Here's how the part is built. I have some questions about the finished solid (model axes, mm). Face numbers are marked on the shaded views. A direction names the side the tool comes from. Give positions to 0.01 mm unless a question says otherwise; leave off trailing zeros. Loops run counter-clockwise (first coordinate to the right, second up) from the corner with the lowest first, then second, coordinate; pieces in that order, holes last. Notation, with made-up numbers: (-22.75, -9.75) - (-7.75, -9.75) arc R33 cw to (-7.75, 18.25) - close; hole circle Ø9 at (-25.75, 85.5). An arc over 180 degrees is marked (long way). Use one line per item in the form item = value.
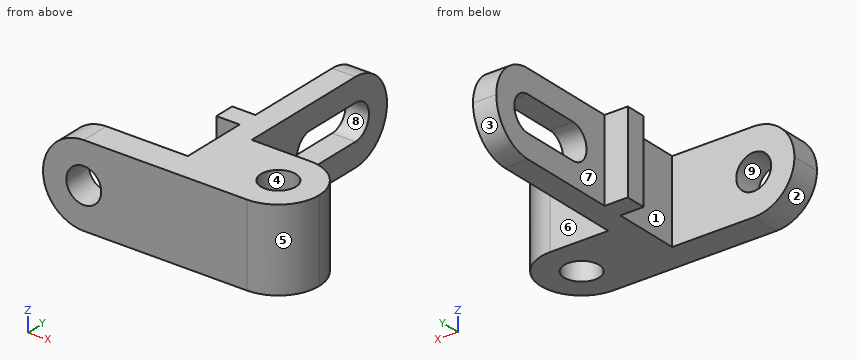
from build123d import *

# Parameters (mm, degrees)
SKETCH2_R           = 6
BOSS_EXTRUDE1_DEPTH = 14
CUT_EXTRUDE1_DEPTH  = 8
SKETCH4_R           = 6
CUT_EXTRUDE2_DEPTH  = 10
FILLET1_R           = 14


with BuildPart() as part:
    # Sketch2 → Boss-Extrude1 (new, symmetric)
    with BuildSketch(Plane.XY):
        Polygon((0, 0), (0, 28), (-34, 28), (-34, 88), (-42, 88), (-42, 40), (-50, 40), (-50, 33), (-42, 33), (-42, 10), (-84, 10), (-84, 0), align=None)
        with Locations((-14, 14)):
            Circle(SKETCH2_R, mode=Mode.SUBTRACT)
    extrude(amount=BOSS_EXTRUDE1_DEPTH, both=True)

    # Sketch3 → Cut-Extrude1 (cut)
    with BuildSketch(Plane(origin=(-34, 0, 0), x_dir=(0, 0, -1), z_dir=(1, 0, 0))):
        with BuildLine():
            Line((-6, 54), (-6, 74))
            ThreePointArc((-6, 74), (0, 80), (6, 74))
            Line((6, 74), (6, 54))
            ThreePointArc((6, 54), (0, 48), (-6, 54))
        make_face()
    extrude(amount=-CUT_EXTRUDE1_DEPTH, mode=Mode.SUBTRACT)

    # Sketch4 → Cut-Extrude2 (cut)
    with BuildSketch(Plane(origin=(0, 10, 0), x_dir=(1, 0, 0), z_dir=(0, 1, 0))):
        with Locations(Location((-70, 0, 0), (0, 0, 180))):
            Circle(SKETCH4_R)
    extrude(amount=-CUT_EXTRUDE2_DEPTH, mode=Mode.SUBTRACT)

    # Fillet1
    fillet1_edges = [part.edges().sort_by_distance(p)[0] for p in [
        (-84, 5, -14),
        (-84, 5, 14),
        (-38, 88, -14),
        (-38, 88, 14),
        (0, 0, 0),
        (0, 28, 0),
    ]]
    fillet(fillet1_edges, radius=FILLET1_R - 0.0001)  # a hair under: the kernel refuses the full size


solid = part.part
(1) If we section it at C-C (x = -18.5): List the corners of the cut face in (y, z) for me.
Geometry says:
outline = (0, -14) - (10.03, -14) - (10.03, 14) - (0, 14) - close; (17.97, -14) - (28, -14) - (28, 14) - (17.97, 14) - close
(2) If we section it at D-D (x = -51.5): List the corners of the cut face in (y, z) for me, plus the area to 3 significant figures.
Geometry says:
outline = (0, -14) - (10, -14) - (10, 14) - (0, 14) - close
area = 280 mm²
(3) For P1, Ø2.5, axis at x = -44, z = -4.5, coming from the +Y side; P2, Ø12, axis at y = 23, z = -9.5, coming from the +X side; P3, Ø1, axis at x = -59.5, z = -3.5, coming from the +Y side, each with a flat end and sliding along its axis, tell me the tip position at first contact or that it passes through.
Geometry says:
P1 = 40
P2 = -0.33
P3 = 10
(4) If we section it at A-A (z = 1.25): Give the number of separate pieces and of enclosed holes in the cut face, plus the area to 3 significant figures.
Geometry says:
separate_pieces = 3
enclosed_holes = 1
area = 1,560 mm²
(5) If we section it at B-B (y = 69.5): List the corners of the cut face in (x, z) for me, plus the area to 3 significant figures.
Geometry says:
outline = (-42, -14) - (-34, -14) - (-34, -6) - (-42, -6) - close; (-42, 6) - (-34, 6) - (-34, 14) - (-42, 14) - close
area = 128 mm²
(6) Thinking about a two-plate mould opening in Y: for the marked faces 1, 2, 3 and 4, which applies, pulls with the +Y half, pulls with the -Y half, needs draft (parallel to the pull), parting line crosses it, or undercut?
Geometry says:
face_1 = undercut
face_2 = needs draft
face_3 = pulls with the +Y half
face_4 = undercut
(7) If I drill on probe 1 along Z at (x, y) = (-37, 59); probe 2 along Y at (x, z) = (-59.5, -1.25); probe 3 along Y at (x, z) = (-14, -2.75), over which ranges is the centre line in solid material (lowest first)?
Geometry says:
probe_1 = -14 to -6, 6 to 14
probe_2 = 0 to 10
probe_3 = 0 to 8, 20 to 28
(8) For the marked faces 5, 6, 7, 8 and 9, which set-ups out of +Z, -Z, +X, -X, +Y, -Y let a thin tool reach every point of the face, with its end or its side?
Geometry says:
face_5 = +Z, -Z, +X, -Y
face_6 = +Z, -Z, +X, +Y
face_7 = +Z, -Z, -X, +Y
face_8 = +X, -X
face_9 = +Y, -Y
